```python
from build123d import *

# Parameters (mm, degrees)
SKETCH1_W               = 120
SKETCH1_H               = 50
BOSS_EXTRUDE1_DEPTH     = 8
SKETCH2_R               = 2.5
CUT_EXTRUDE1_DEPTH      = 10
MIRROR2_COPY_1_SKETCH_R = 2.5
MIRROR2_COPY_1_DEPTH    = 10
SKETCH4_W               = 5
SKETCH4_H               = 20
BOSS_EXTRUDE2_DEPTH     = 15
FILLET1_R               = 5
FILLET1_OF_MIRROR4_R    = 5
SKETCH5_R               = 2.5
CUT_EXTRUDE2_DEPTH      = 54


with BuildPart() as part:
    # Sketch1 → Boss-Extrude1 (new body)
    with BuildSketch(Plane(origin=(0, 0, 0), x_dir=(1, 0, 0), z_dir=(0, 1, 0))):
        with BuildLine():
            Line((-80, 60), (80, 60))
            ThreePointArc((80, 60), (94.142135624, 54.142135624), (100, 40))
            Line((100, 40), (100, -40))
            ThreePointArc((100, -40), (94.142135624, -54.142135624), (80, -60))
            Line((80, -60), (-80, -60))
            ThreePointArc((-80, -60), (-94.142135624, -54.142135624), (-100, -40))
            Line((-100, -40), (-100, 40))
            ThreePointArc((-100, 40), (-94.142135624, 54.142135624), (-80, 60))
        make_face()
        Rectangle(SKETCH1_W, SKETCH1_H, mode=Mode.SUBTRACT)
    extrude(amount=BOSS_EXTRUDE1_DEPTH)

    # Sketch2 → Cut-Extrude1 (cut)
    with BuildSketch(Plane(origin=(0, 8, 0), x_dir=(1, 0, 0), z_dir=(0, 1, 0))):
        with Locations(Location((85, -45, 0), (0, 0, 270))):
            Circle(SKETCH2_R)
    cut_extrude1 = extrude(amount=-CUT_EXTRUDE1_DEPTH, mode=Mode.SUBTRACT)

    # Mirror1: Cut-Extrude1 across plane
    add(cut_extrude1.mirror(Plane(origin=(0, 0, 0), x_dir=(0, 0, 1), z_dir=(1, 0, 0))), mode=Mode.SUBTRACT)

    # Mirror2: Cut-Extrude1 across plane
    add(cut_extrude1.mirror(Plane.XY), mode=Mode.SUBTRACT)

    # Mirror2 copy 1 sketch → Mirror2 copy 1 (cut)
    with BuildSketch(Plane(origin=(0, 8, 0), x_dir=(-1, 0, 0), z_dir=(0, 1, 0))):
        with Locations(Location((85, -45, 0), (0, 0, 270))):
            Circle(MIRROR2_COPY_1_SKETCH_R)
    extrude(amount=-MIRROR2_COPY_1_DEPTH, mode=Mode.SUBTRACT)

    # Sketch4 → Boss-Extrude2 (add)
    with BuildSketch(Plane(origin=(0, 8, 0), x_dir=(1, 0, 0), z_dir=(0, 1, 0))):
        with Locations((10, 45)):
            Rectangle(SKETCH4_W, SKETCH4_H)
    boss_extrude2 = extrude(amount=BOSS_EXTRUDE2_DEPTH)

    # Fillet1
    fillet1_edges = [part.edges().sort_by_distance(p)[0] for p in [
        (10, 23, -55),
        (10, 23, -35),
    ]]
    fillet(fillet1_edges, radius=FILLET1_R)

    # Mirror4: Boss-Extrude2 across plane
    add(boss_extrude2.mirror(Plane(origin=(0, 0, 0), x_dir=(0, 0, 1), z_dir=(1, 0, 0))))

    # Fillet1 of Mirror4
    fillet1_of_mirror4_edges = [part.edges().sort_by_distance(p)[0] for p in [
        (-10, 23, -55),
        (-10, 23, -35),
    ]]
    fillet(fillet1_of_mirror4_edges, radius=FILLET1_OF_MIRROR4_R)

    # Sketch5 → Cut-Extrude2 (cut)
    with BuildSketch(Plane(origin=(12.5, 0, 0), x_dir=(0, 0, -1), z_dir=(1, 0, 0))):
        with Locations((45, 18)):
            Circle(SKETCH5_R)
    extrude(amount=-CUT_EXTRUDE2_DEPTH, mode=Mode.SUBTRACT)


solid = part.part
```
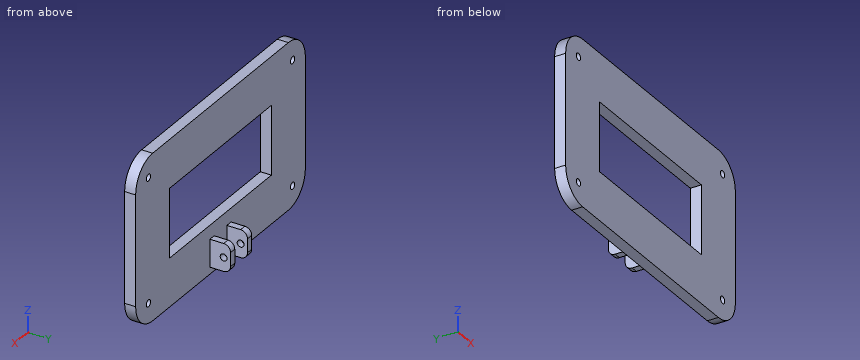
Geometry: final body of the model. Coordinates: model frame, mm. Coordinates: 2 decimals unless noted, no trailing zeros. Order: outer loops, then holes, each group sorted by start corner. A loop starts at its lowest first (then second) coordinate and runs counter-clockwise, first axis right, second up. Notation, with made-up numbers: M -24.75,31.25 L -5.75,31.25 A23 cw -5.75,70.25 Z; hole C 56.5,44.5 d5. An arc over 180 degrees is marked long. Answer as CSV lines item,"result".
Q1. Line query: probe 1 along X at (y, z) = (3, -4.5); probe 2 along Z at (x, y) = (-85, 3.25); probe 3 along Z at (x, y) = (19, 3.5). Output: solid intervals per line, ascending. Write a range as [from, to].
Answers:
probe 1,"x = [-100, -60], [60, 100]"
probe 2,"z = [-59.36, -47.5], [-42.5, 42.5], [47.5, 59.36]"
probe 3,"z = [-60, -25], [25, 60]"
Q2. First-contact query: P1, Ø10, axis at x = 17, y = 17.5, coming from the +Z side; P2, Ø4, axis at x = 10.5, y = 10.5, coming from the -Z side; P3, Ø4.5, axis at y = 18, z = -48.5, coming from the -X side; P4, Ø4, axis at x = -85, z = -45, coming from the +Y side. Flat tips, straight axial feed; report the tip coordinate or a pass-through.
Answers:
P1,"stops at z = -35"
P2,"stops at z = -55"
P3,"stops at x = -12.5"
P4,"passes through"
Q3. Section B-B on x = -49.5. Return the cut outline in (y, z).
Answers:
outline,"M 0,-60 L 8,-60 L 8,-25 L 0,-25 Z; M 0,25 L 8,25 L 8,60 L 0,60 Z"
Q4. Section C-C on x = -85. Return the cut outline in (y, z), and give its area (3 significant figures).
Answers:
outline,"M 0,-59.36 L 8,-59.36 L 8,-47.5 L 0,-47.5 Z; M 0,-42.5 L 8,-42.5 L 8,42.5 L 0,42.5 Z; M 0,47.5 L 8,47.5 L 8,59.36 L 0,59.36 Z"
area,"870 mm^2"
Q5. Section A-A on z = -17.5. Return the cut outline in (x, y), and give its area (3 significant figures).
Answers:
outline,"M -100,0 L -60,0 L -60,8 L -100,8 Z; M 60,0 L 100,0 L 100,8 L 60,8 Z"
area,"640 mm^2"
Q6. Section D-D on z = -45. Return the cut outline in (x, y).
Answers:
outline,"M -99.36,0 L -87.5,0 L -87.5,8 L -99.36,8 Z; M -82.5,0 L 82.5,0 L 82.5,8 L 12.5,8 L 12.5,15.5 L 7.5,15.5 L 7.5,8 L -7.5,8 L -7.5,15.5 L -12.5,15.5 L -12.5,8 L -82.5,8 Z; M -12.5,20.5 L -7.5,20.5 L -7.5,23 L -12.5,23 Z; M 7.5,20.5 L 12.5,20.5 L 12.5,23 L 7.5,23 Z; M 87.5,0 L 99.36,0 L 99.36,8 L 87.5,8 Z"
